Answer from the drawing. Dimensions are ordinates in mm from the lowest x, y and z of the part. A direction names the side the tool comes from. Give positions to 0.01 mm unless a question says otherwise; leave off trailing zeros. Loops run counter-clockwise (first coordinate to the right, second up) from the corner with the lowest first, then second, coordinate; pieces in that order, holes last.
(1) Find section B-B, the plane y = 29.5. Write down the section's boundary in (x, z).
(2) Each of these flat-tipped pins is pushed along its axis until it touches: P1, Ø3, axis at y = 30, z = 38, coming from the +X side; P2, Ø24, axis at x = 32.5, y = 32.5, coming from the +Z side; P3, Ø24, axis at x = 24, y = 50, coming from the -Z side; P4, Ø1.5, axis at x = 50.5, z = 41, coming from the -Y side. Where does it stop, or does it pass through?
(3) Which of the six approach directions +Z, -Z, +X, -X, +Y, -Y give full straight-line access (tool end or side, diameter ignored) to the marked faces 1, 2, 3, 4 and 5?
(4) Find section A-A, the plane y = 48. Write down the section's boundary in (x, z) (3 decimals), then the cut area to 3 significant figures.
(5) Determine the mould class of the marked faces 6, 7 and 8 for opening direction Y: pulls with the +Y half, pulls with the -Y half, needs draft (parallel to the pull), parting line crosses it, or undercut.
(6) Find section D-D, the plane x = 15. Write down the section's boundary in (y, z), then the cut area to 3 significant figures.
(7) Straight lines are drawn through the part: probe 1 along X at (y, z) = (3.1, 54); probe 2 along Z at (x, y) = (48, 2); probe 3 along Y at (x, z) = (3.6, 23) (3 decimals). For each, find the intervals that lie inside material, in ascending order.
(8) Find section C-C, the plane z = 39. Write down the section's boundary in (x, y) (3 decimals), then the cut area to 3 significant figures.
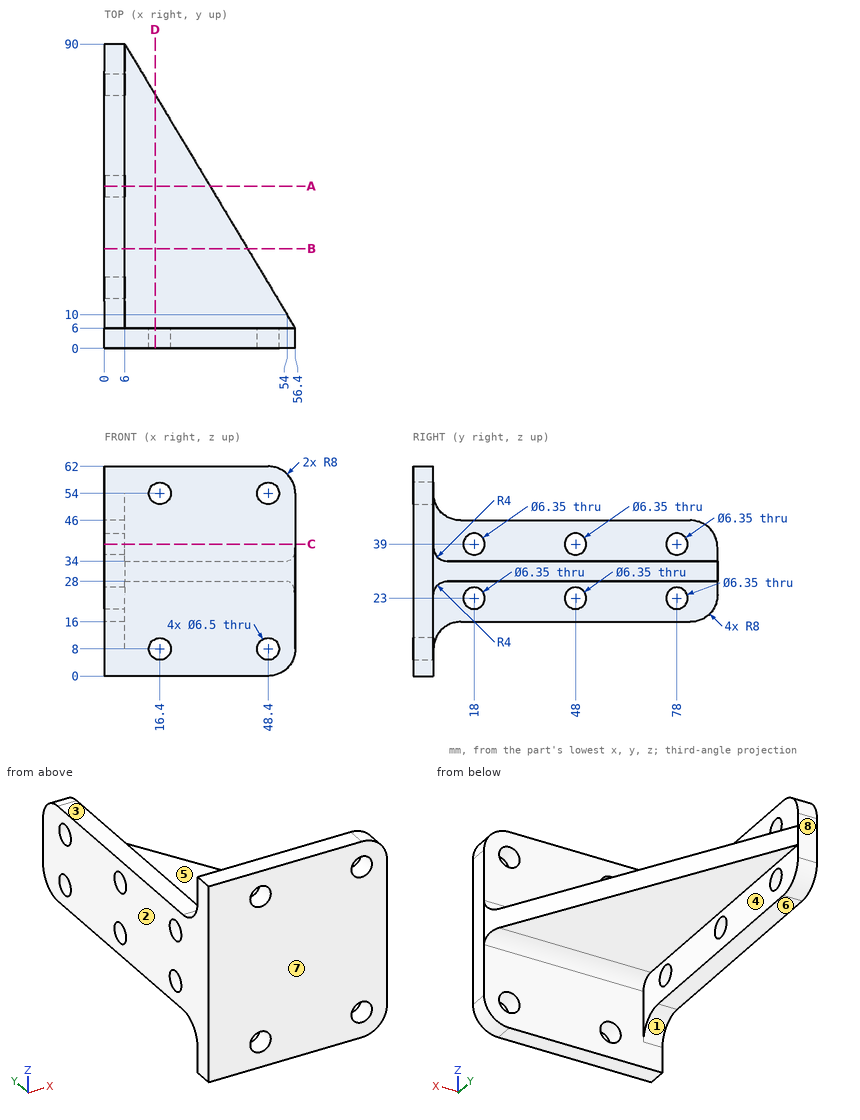
Entries:
1. outline: (0, 16) - (6, 16) - (6, 28) - (42.3, 28) - (42.3, 34) - (6, 34) - (6, 46) - (0, 46) - close
2. P1: stops at x = 6
2. P2: stops at z = 34
2. P3: stops at z = 28
2. P4: stops at y = 0
3. face 1: -Z, +X, -X, +Y
3. face 2: +Z, -Z, -X, +Y, -Y
3. face 3: +Z, +X, -X, +Y
3. face 4: -Z, +X, +Y
3. face 5: +Z, +X, +Y
4. outline: (0, 16) - (6, 16) - (6, 19.825) - (0, 19.825) - close; (0, 26.175) - (6, 26.175) - (6, 28) - (31.2, 28) - (31.2, 34) - (6, 34) - (6, 35.825) - (0, 35.825) - close; (0, 42.175) - (6, 42.175) - (6, 46) - (0, 46) - close
4. area: 255 mm2
5. face 6: needs draft
5. face 7: pulls with the -Y half
5. face 8: pulls with the +Y half
6. outline: (0, 0) - (6, 0) - (6, 5.07) - (0, 5.07) - close; (0, 10.93) - (6, 10.93) - (6, 24) arc R4 cw to (10, 28) - (75, 28) - (75, 34) - (10, 34) arc R4 cw to (6, 38) - (6, 51.07) - (0, 51.07) - close; (0, 56.93) - (6, 56.93) - (6, 62) - (0, 62) - close
6. area: 722 mm2
7. probe 1: x = 0 to 13.15, 19.65 to 45.15, 51.65 to 56.4
7. probe 2: z = 0 to 4.77, 11.23 to 50.77, 57.23 to 62
7. probe 3: y = 0 to 14.825, 21.175 to 44.825, 51.175 to 74.825, 81.175 to 89.937
8. outline: (0, 0) - (56.4, 0) - (56.4, 6) - (6, 6) - (6, 14.825) - (0, 14.825) - close; (0, 21.175) - (6, 21.175) - (6, 44.825) - (0, 44.825) - close; (0, 51.175) - (6, 51.175) - (6, 74.825) - (0, 74.825) - close; (0, 81.175) - (6, 81.175) - (6, 89.937) - (0, 89.937) - close
8. area: 728 mm2
